The model under review builds one solid part; all positions refer to its coordinate system, in mm. Face numbers are marked on the shaded views. A direction names the side the tool comes from. Coordinates: 2 decimals unless noted, no trailing zeros. Write each loop counter-clockwise with the first axis right and the second up, starting at its lowest first coordinate (ties: lowest second). Pieces come first, ordered by that corner, then holes. Notation, with made-up numbers: (-16.5, 10.5) - (-0.5, 10.5) arc R19 ccw to (-0.5, 26.5) - close; hole circle Ø9 at (73.5, 88.5). An arc over 180 degrees is marked (long way). Answer as CSV lines item,"result". Start each with the question number.
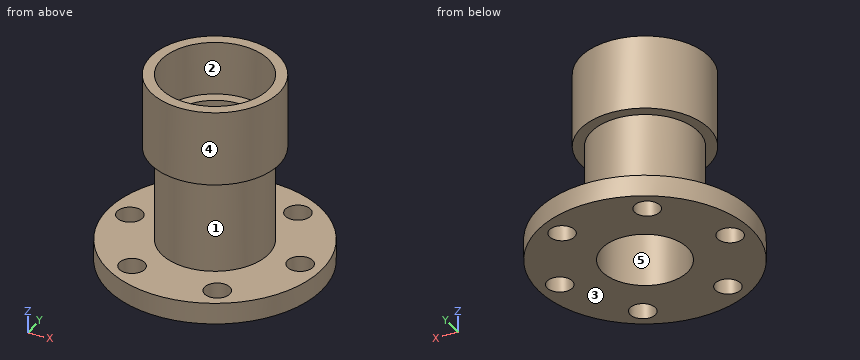
```python
from build123d import *

# Parameters (mm, degrees)
SKETCH2_R          = 5.9
CUT_EXTRUDE1_DEPTH = 10


with BuildPart() as part:
    # Sketch1 → Revolve1 (revolve)
    with BuildSketch(Plane(origin=(0, 0, 0), x_dir=(0, 0, -1), z_dir=(1, 0, 0)), mode=Mode.PRIVATE) as revolve1_sk:
        Polygon((0, 20), (0, 50), (-10, 50), (-10, 25), (-55, 25), (-55, 30), (-90, 30), (-90, 25), (-65, 25), (-65, 20), align=None)
    revolve(revolve1_sk.sketch.rotate(Axis((0, 0, 0), (0, 0, 1)), 90), axis=Axis((0, 0, 0), (0, 0, 1)))

    # Sketch2 → Cut-Extrude1 (cut)
    with BuildSketch(Plane.XY.offset(10)):
        with Locations((40, 0)):
            Circle(SKETCH2_R)
        with Locations((20, -34.641016151)):
            Circle(SKETCH2_R)
        with Locations((-20, -34.641016151)):
            Circle(SKETCH2_R)
        with Locations((-40, 0)):
            Circle(SKETCH2_R)
        with Locations((-20, 34.641016151)):
            Circle(SKETCH2_R)
        with Locations((20, 34.641016151)):
            Circle(SKETCH2_R)
    extrude(amount=-CUT_EXTRUDE1_DEPTH, mode=Mode.SUBTRACT)


solid = part.part
```
(1) Add section A-A on x = 0. Give the boundary of the cut face in (y, z).
(2) For pin 1 (13.5 mm diameter, centred on x = -20, y = -34.64, fed in from +Z); pin 2 (4 mm diameter, centred on y = -18.5, z = 34, fed in from -X); pin 3 (5 mm diameter, centred on y = 0.5, z = 32, fed in from +X), all flat-tipped, find the tip position at first contact; note any pin that passes through.
(3) For the marked faces 4 and 5, list the 3-axis set-ups (+Z, -Z, +X, -X, +Y, -Y) from which the entire face can be reached by the end or side of a thin tool; tool diameter is ignored.
(4) The part is to be moulded in two halves that separate along Z. For the marked faces 1, 2 and 3, say which applies: released by +Z, released by -Z, zero draft, split by the parting line, or undercut.
(5) Wall thickness on line 1 (Y direction, x = 40, z = 3); line 2 (X direction, y = 0.5, z = 75.5) (3 decimals); line 3 (Z direction, x = -27, y = 12): over which ranges is each line inside the solid? List them lowest first.
(6) Add section C-C on y = 37. Give the boundary of the cut face in (x, z).
(7) Add section D-D on y = -4. Give the boundary of the cut face in (x, z).
(8) Add section B-B on z = 19. Give the boundary of the cut face in (x, y).
Reported:
1,outline,"(-50, 0) - (-20, 0) - (-20, 65) - (-25, 65) - (-25, 90) - (-30, 90) - (-30, 55) - (-25, 55) - (-25, 10) - (-50, 10) - close; (20, 0) - (50, 0) - (50, 10) - (25, 10) - (25, 55) - (30, 55) - (30, 90) - (25, 90) - (25, 65) - (20, 65) - close"
2,pin 1,"z = 10"
2,pin 2,"x = -18.78"
2,pin 3,"x = 25"
3,face 4,"+Z"
3,face 5,"+Z, -Z"
4,face 1,"undercut"
4,face 2,"zero draft"
4,face 3,"released by -Z"
5,line 1,"-30 to -5.9, 5.9 to 30"
5,line 2,"-29.996 to -24.995, 24.995 to 29.996"
5,line 3,"0 to 10, 55 to 90"
6,outline,"(-33.63, 0) - (-25.41, 0) - (-25.41, 10) - (-33.63, 10) - close; (-14.59, 0) - (14.59, 0) - (14.59, 10) - (-14.59, 10) - close; (25.41, 0) - (33.63, 0) - (33.63, 10) - (25.41, 10) - close"
7,outline,"(-49.84, 0) - (-44.34, 0) - (-44.34, 10) - (-49.84, 10) - close; (-35.66, 0) - (-19.6, 0) - (-19.6, 65) - (-24.68, 65) - (-24.68, 90) - (-29.73, 90) - (-29.73, 55) - (-24.68, 55) - (-24.68, 10) - (-35.66, 10) - close; (19.6, 0) - (35.66, 0) - (35.66, 10) - (24.68, 10) - (24.68, 55) - (29.73, 55) - (29.73, 90) - (24.68, 90) - (24.68, 65) - (19.6, 65) - close; (44.34, 0) - (49.84, 0) - (49.84, 10) - (44.34, 10) - close"
8,outline,"circle Ø50 at (0, 0); hole circle Ø40 at (0, 0)"
